Model file for the job. Use its own axes, mm. Face numbers are marked on the shaded views. Give positions to 0.01 mm unless a question says otherwise; leave off trailing zeros. Loops run counter-clockwise (first coordinate to the right, second up) from the corner with the lowest first, then second, coordinate; pieces in that order, holes last. Notation, with made-up numbers: M 87,72.25 L 137,72.25 A19 ccw 137,101.25 Z; hole C 60.5,-10 d4. An arc over 180 degrees is marked long. Answer in a Markdown table with one row per item.
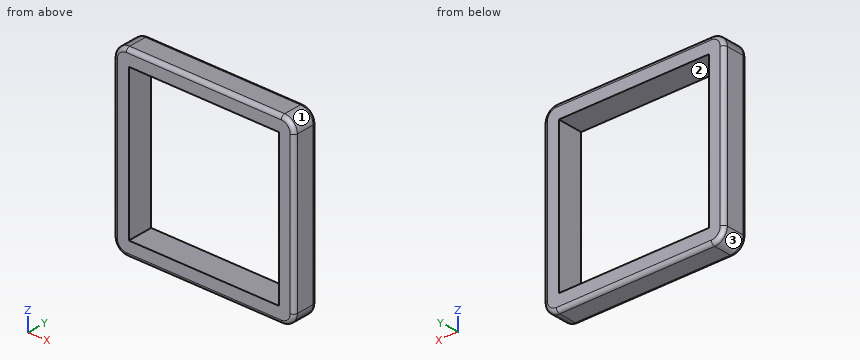
```python
from build123d import *

# Parameters (mm, degrees)
SKETCH1_W           = 901.7
SKETCH1_H           = 901.7
SKETCH1_W_2         = 749.3
SKETCH1_H_2         = 749.3
BOSS_EXTRUDE1_DEPTH = 127
FILLET1_R           = 63.5
FILLET2_R           = 19.05


with BuildPart() as part:
    # Sketch1 → Boss-Extrude1 (new body)
    with BuildSketch(Plane(origin=(0, 0, 0), x_dir=(1, 0, 0), z_dir=(0, 1, 0))):
        Rectangle(SKETCH1_W, SKETCH1_H)
        Rectangle(SKETCH1_W_2, SKETCH1_H_2, mode=Mode.SUBTRACT)
    extrude(amount=BOSS_EXTRUDE1_DEPTH)

    # Fillet1
    fillet1_edges = [part.edges().sort_by_distance(p)[0] for p in [
        (-450.85, 63.5, -450.85),
        (450.85, 63.5, -450.85),
        (450.85, 63.5, 450.85),
        (-450.85, 63.5, 450.85),
    ]]
    fillet(fillet1_edges, radius=FILLET1_R)

    # Fillet2
    fillet2_edges = [part.edges().sort_by_distance(p)[0] for p in [
        (-450.85, 0, 0),
        (-450.85, 127, 0),
        (0, 0, -450.85),
        (450.85, 0, 0),
        (0, 0, 450.85),
        (-432.251280605, 0, 432.251280605),
        (432.251280605, 0, 432.251280605),
        (432.251280605, 0, -432.251280605),
        (-432.251280605, 0, -432.251280605),
        (0, 127, -450.85),
        (0, 127, 450.85),
        (450.85, 127, 0),
        (-432.251280605, 127, 432.251280605),
        (432.251280605, 127, 432.251280605),
        (432.251280605, 127, -432.251280605),
        (-432.251280605, 127, -432.251280605),
    ]]
    fillet(fillet2_edges, radius=FILLET2_R)


solid = part.part
```
Q1. Saw through at A-A (z = -316). Give the cut face in (x, y), and give its area (3 significant figures).
Reported:
| item | result |
|---|---|
| outline | M -450.85,19.05 A19.05 ccw -431.8,0 L -374.65,0 L -374.65,127 L -431.8,127 A19.05 ccw -450.85,107.95 Z; M 374.65,0 L 431.8,0 A19.05 ccw 450.85,19.05 L 450.85,107.95 A19.05 ccw 431.8,127 L 374.65,127 Z |
| area | 19,000 mm² |
Q2. Drop flat-ended pins along their axis: pin 1 (1.5 mm diameter, centred on y = 13.5, z = -155, fed in from +X); pin 2 (1 mm diameter, centred on x = -229.5, y = 14.5, fed in from +Z). Give the stop position or say it passes through.
Reported:
| item | result |
|---|---|
| pin 1 | x = 450.24 |
| pin 2 | z = 450.41 |
Q3. Saw through at C-C (y = 80). Give the cut face in (x, z), and give its area (3 significant figures).
Reported:
| item | result |
|---|---|
| outline | M -450.85,-387.35 A63.5 ccw -387.35,-450.85 L 387.35,-450.85 A63.5 ccw 450.85,-387.35 L 450.85,387.35 A63.5 ccw 387.35,450.85 L -387.35,450.85 A63.5 ccw -450.85,387.35 Z; hole M -374.65,-374.65 L 374.65,-374.65 L 374.65,374.65 L -374.65,374.65 Z |
| area | 248,000 mm² |
Q4. Saw through at B-B (x = 96.5). Give the cut face in (y, z), and give its area (3 significant figures).
Reported:
| item | result |
|---|---|
| outline | M 0,-431.8 A19.05 ccw 19.05,-450.85 L 107.95,-450.85 A19.05 ccw 127,-431.8 L 127,-374.65 L 0,-374.65 Z; M 0,374.65 L 127,374.65 L 127,431.8 A19.05 ccw 107.95,450.85 L 19.05,450.85 A19.05 ccw 0,431.8 Z |
| area | 19,000 mm² |
Q5. Mould opens along Z. For the marked faces 1, 2 and 3 say: released by +Z, released by -Z, zero draft, split by the parting line, or undercut.
Reported:
| item | result |
|---|---|
| face 1 | released by +Z |
| face 2 | undercut |
| face 3 | released by -Z |
Q6. Probe probe 1 along Z at (x, y) = (-206, 101.5); probe 2 along Z at (x, y) = (317.5, 120). List the from-to ranges inside material, lowest first.
Reported:
| item | result |
|---|---|
| probe 1 | -450.85 to -374.65, 374.65 to 450.85 |
| probe 2 | -446.55 to -374.65, 374.65 to 446.55 |
